For this review, take the finished solid that the model builds, in its own axes (mm). Face numbers are marked on the shaded views. A direction names the side the tool comes from. Round coordinates to 2 decimals unless told otherwise and drop trailing zeros. Write each loop counter-clockwise with the first axis right and the second up, starting at its lowest first coordinate (ties: lowest second). Pieces come first, ordered by that corner, then holes.
from build123d import *

# Parameters (mm, degrees)
SKETCH_1_W      = 27
SKETCH_1_H      = 27
SKETCH_1_R      = 1.6
EXTRUDE_1_DEPTH = 2
SKETCH_2_R      = 7.5
EXTRUDE_2_DEPTH = 20
SKETCH_3_W      = 16
SKETCH_3_H      = 15
EXTRUDE_3_DEPTH = 8
SKETCH_4_W      = 3.5
SKETCH_4_H      = 22
EXTRUDE_4_DEPTH = 10


with BuildPart() as part:
    # 草图1 → 凸台-拉伸1 (new body)
    with BuildSketch(Plane.XY):
        with Locations((255, 320)):
            Rectangle(SKETCH_1_W, SKETCH_1_H)
        with Locations((266.5, 331.5)):
            Circle(SKETCH_1_R, mode=Mode.SUBTRACT)
        with Locations((266.5, 308.5)):
            Circle(SKETCH_1_R, mode=Mode.SUBTRACT)
    extrude(amount=EXTRUDE_1_DEPTH)

    # 草图2 → 凸台-拉伸2 (add)
    with BuildSketch(Plane.XY.offset(2)):
        with Locations((260, 320)):
            Circle(SKETCH_2_R)
    extrude(amount=EXTRUDE_2_DEPTH)

    # 草图3 → 凸台-拉伸3 (add)
    with BuildSketch(Plane.XY.offset(2)):
        with Locations((260.5, 320)):
            Rectangle(SKETCH_3_W, SKETCH_3_H)
    extrude(amount=EXTRUDE_3_DEPTH)

    # 草图4 → 凸台-拉伸4 (add)
    with BuildSketch(Plane(origin=(0, 0, 0), x_dir=(-1, 0, 0), z_dir=(0, 0, -1))):
        with Locations((-243.92, 320)):
            Rectangle(SKETCH_4_W, SKETCH_4_H)
    extrude(amount=EXTRUDE_4_DEPTH)


solid = part.part
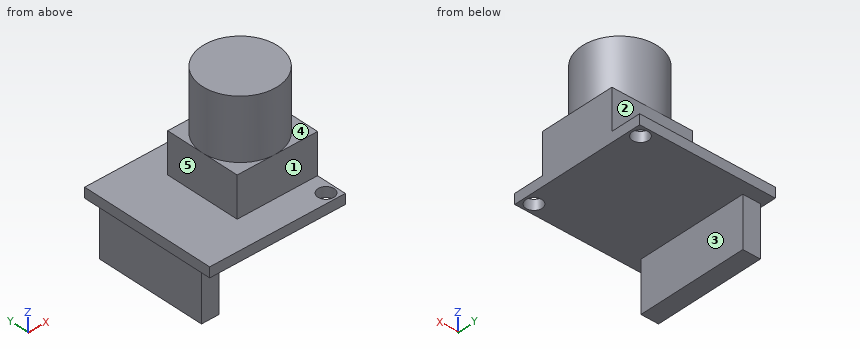
(1) For the marked faces 1, 2, 3, 4 and 5, list the 3-axis set-ups (+Z, -Z, +X, -X, +Y, -Y) from which the entire face can be reached by the end or side of a thin tool; tool diameter is ignored.
Geometry check:
face 1: +Z, +X, -X, -Y
face 2: +Z, +X, -X, +Y
face 3: -Z, +X, +Y, -Y
face 4: +Z, +X
face 5: +Z, -X, +Y, -Y
(2) We need section C-C, the plane z = 0.5. Give the boundary of the cut face in (x, y), and give its area (3 significant figures).
Geometry check:
outline: (241.5, 306.5) - (268.5, 306.5) - (268.5, 333.5) - (241.5, 333.5) - close; hole circle Ø3.2 at (266.5, 308.5); hole circle Ø3.2 at (266.5, 331.5)
area: 713 mm2
(3) For pin 1 Ø3 at (x, y) = (266.5, 308.5) entering from +Z; pin 2 Ø1 at (x, z) = (243.5, -6) entering from +Y; pin 3 Ø5 at (y, z) = (319.5, -5) entering from -X; pin 4 Ø6 at (x, z) = (252, 12.5) entering from +Y, all flat-tipped, find the tip position at first contact; note any pin that passes through.
Geometry check:
pin 1: passes through
pin 2: stops at y = 331
pin 3: stops at x = 242.17
pin 4: stops at y = 327.5
(4) For line 1 along Y through (x, z) = (266.5, 1.15); line 2 along X through (y, z) = (308.5, 1.45); line 3 along Z through (x, y) = (257, 315.5), list the stretches that pass through material, from the lowest coordinate up.
Geometry check:
line 1: y = 306.5 to 306.9, 310.1 to 329.9, 333.1 to 333.5
line 2: x = 241.5 to 264.9, 268.1 to 268.5
line 3: z = 0 to 22
(5) We need section D-D, the plane x = 253. Give the boundary of the cut face in (y, z).
Geometry check:
outline: (306.5, 0) - (333.5, 0) - (333.5, 2) - (327.5, 2) - (327.5, 10) - (322.69, 10) - (322.69, 22) - (317.31, 22) - (317.31, 10) - (312.5, 10) - (312.5, 2) - (306.5, 2) - close
(6) We need section B-B, the plane x = 266.5. Give the boundary of the cut face in (y, z).
Geometry check:
outline: (306.5, 0) - (306.9, 0) - (306.9, 2) - (306.5, 2) - close; (310.1, 0) - (329.9, 0) - (329.9, 2) - (327.5, 2) - (327.5, 10) - (323.74, 10) - (323.74, 22) - (316.26, 22) - (316.26, 10) - (312.5, 10) - (312.5, 2) - (310.1, 2) - close; (333.1, 0) - (333.5, 0) - (333.5, 2) - (333.1, 2) - close
(7) We need section A-A, the plane y = 331.5. Give the boundary of the cut face in (x, z), and give its area (3 significant figures).
Geometry check:
outline: (241.5, 0) - (264.9, 0) - (264.9, 2) - (241.5, 2) - close; (268.1, 0) - (268.5, 0) - (268.5, 2) - (268.1, 2) - close
area: 47.6 mm2
